Here's the drawing with two shaded views (mm, measured from the low corner). I have some questions. Give positions to 0.01 mm unless a question says otherwise; leave off trailing zeros. Loops run counter-clockwise (first coordinate to the right, second up) from the corner with the lowest first, then second, coordinate; pieces in that order, holes last. Notation, with made-up numbers: (12.5, -16.75) - (67.5, -16.75) arc R11 cw to (67.5, 0.25) - close; hole circle Ø4 at (11.25, -9). An arc over 180 degrees is marked (long way). Write each question's results on one line, items separated by ' | '. Start each with the question number.
1) I'm going to push flat-ended pins straight in: pin 1 (1 mm diameter, centred on y = 5.5, z = 3.5, fed in from -X); pin 2 (2 mm diameter, centred on x = 4, y = 2.5, fed in from -Z). Where does each tip first touch, or does it pass through?
2) If I drill on probe 1 along X at (y, z) = (1.75, 3.5); probe 2 along Y at (x, z) = (3.75, 11.5); probe 3 along X at (y, z) = (4.75, 3.75), over which ranges is the centre line in solid material (lowest first)? Write a range as [from, to].
3) I want a section at A-A, the plane z = 11. Write out the boundary of the cut face in (x, y), and give its area (3 significant figures).
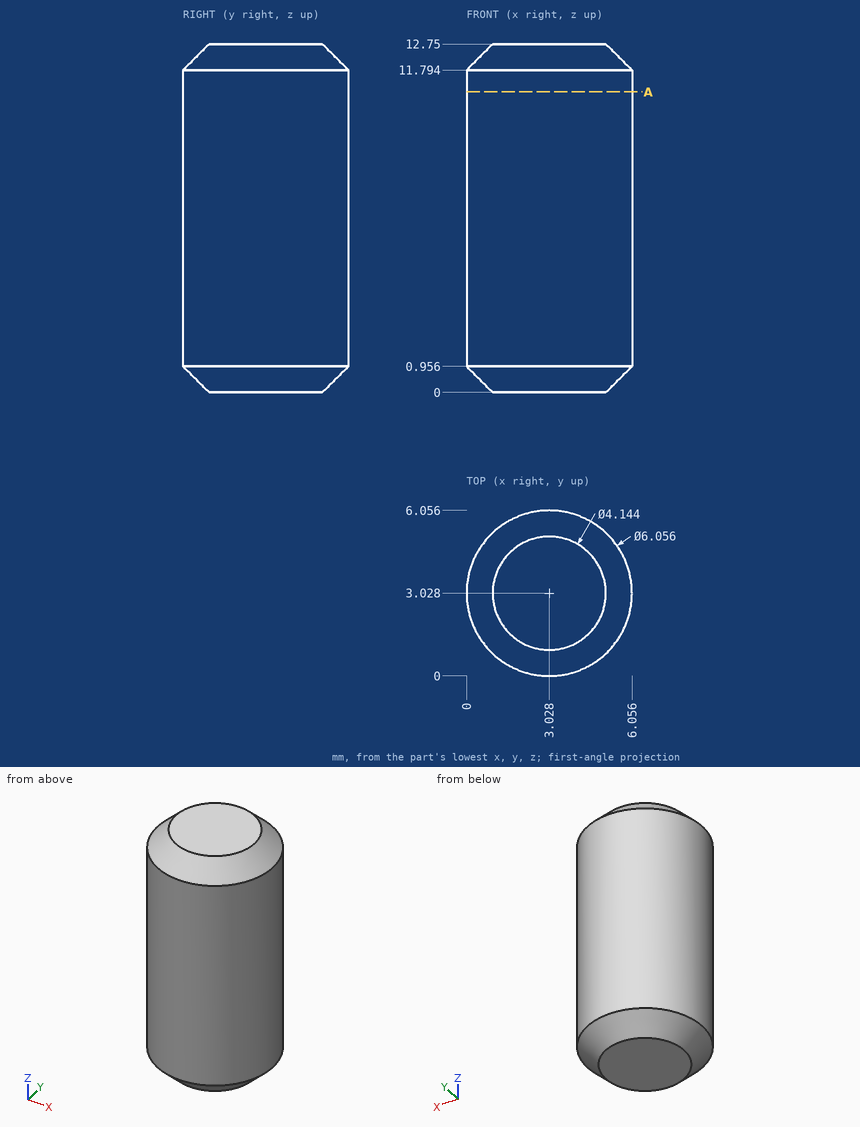
Answers:
1) pin 1: stops at x = 0.73 | pin 2: stops at z = 0
2) probe 1: x = [0.28, 5.77] | probe 2: y = [0.09, 5.97] | probe 3: x = [0.54, 5.52]
3) outline: circle Ø6.06 at (3.03, 3.03) | area: 28.8 mm2
